Answer from the drawing. Dimensions are ordinates in mm from the lowest x, y and z of the part. A direction names the side the tool comes from. Give positions to 0.01 mm unless a question says otherwise; leave off trailing zeros. Order: outer loops, then holes, each group sorted by start corner. A loop starts at its lowest first (then second) coordinate and runs counter-clockwise, first axis right, second up. Notation, with made-up numbers: (69, 27.25) -> (107, 27.25) arc R27 cw to (107, 65.25) -> close; hole circle Ø5 at (8, 79). An arc over 180 degrees is marked (long way). One line per question, with ' | ' between items. Start each with the question number.
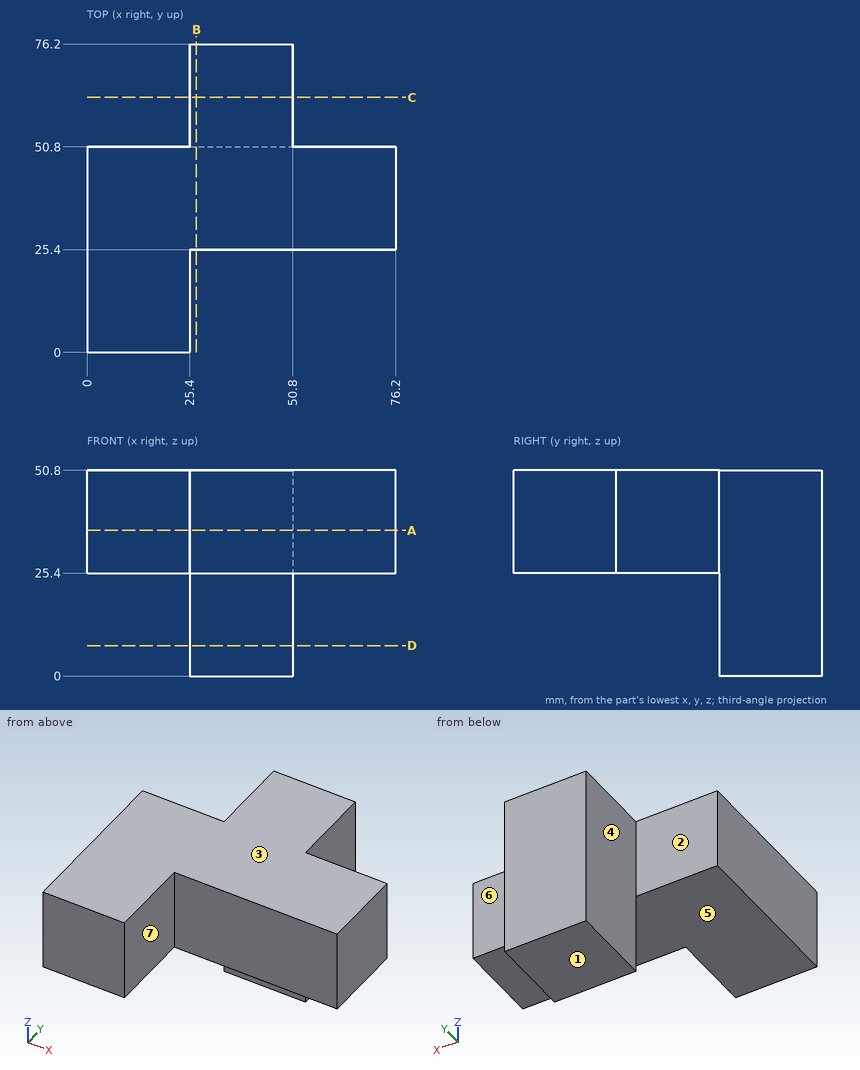
(1) Consider line 1 (X direction, y = 55.5, z = 43.5); line 2 (Y direction, x = 4, z = 35). Determine where each line is inside the solid, lowest interval first.
(2) The part is cut by section D-D on z = 7.5. Determine the outline of the cut face in (x, y).
(3) Given P1, Ø1.5, axis at x = 34.5, z = 19.5, coming from the -Y side; P2, Ø4, axis at x = 65.5, z = 33.5, coming from the +Y side; P3, Ø15, axis at x = 45.5, y = 38, coming from the -Z side; P4, Ø8, axis at x = 24, y = 53.5, coming from the -Z side, each flat-ended and moving along its own axis, determine where each tip first touches the part or whether it passes through.
(4) The part is cut by section A-A on z = 36. Determine the outline of the cut face in (x, y).
(5) The part is cut by section B-B on x = 27. Determine the outline of the cut face in (y, z).
(6) Determine the mould class of the marked faces 1, 2 and 3 for opening direction Z: pulls with the +Z half, pulls with the -Z half, needs draft (parallel to the pull), parting line crosses it, or undercut.
(7) The part is cut by section C-C on y = 63. Determine the outline of the cut face in (x, z).
(8) For the marked faces 4, 5, 6 and 7, determine the directions among +Z, -Z, +X, -X, +Y, -Y from which every point of the face is accessible in a straight line to the end or side of a thin tool.
Result sheet:
1) line 1: x = 25.4 to 50.8 | line 2: y = 0 to 50.8
2) outline: (25.4, 50.8) -> (50.8, 50.8) -> (50.8, 76.2) -> (25.4, 76.2) -> close
3) P1: stops at y = 50.8 | P2: stops at y = 50.8 | P3: stops at z = 25.4 | P4: stops at z = 0
4) outline: (0, 0) -> (25.4, 0) -> (25.4, 25.4) -> (76.2, 25.4) -> (76.2, 50.8) -> (50.8, 50.8) -> (50.8, 76.2) -> (25.4, 76.2) -> (25.4, 50.8) -> (0, 50.8) -> close
5) outline: (25.4, 25.4) -> (50.8, 25.4) -> (50.8, 0) -> (76.2, 0) -> (76.2, 50.8) -> (25.4, 50.8) -> close
6) face 1: pulls with the -Z half | face 2: needs draft | face 3: pulls with the +Z half
7) outline: (25.4, 0) -> (50.8, 0) -> (50.8, 50.8) -> (25.4, 50.8) -> close
8) face 4: +Z, -Z, -X, +Y | face 5: -Z, +X, -X, -Y | face 6: +Z, -Z, +X, +Y | face 7: +Z, -Z, +X, -Y
